The model under review builds one solid part; all positions refer to its coordinate system, in mm. A direction names the side the tool comes from. Give positions to 0.01 mm unless a question says otherwise; leave off trailing zeros. Order: outer loops, then holes, each group sorted by start corner. A loop starts at its lowest first (then second) coordinate and runs counter-clockwise, first axis right, second up. Notation, with made-up numbers: (-3.5, 83) - (48.5, 83) arc R19 ccw to (48.5, 92) - close; hole circle Ø10 at (22, -33). An arc over 180 degrees is marked (long way). Answer as CSV lines item,"result". Start each with the question number.
from build123d import *

# Parameters (mm, degrees)
F0_W     = 5
F0_H     = 95
F1_DEPTH = 1.4
F3_DEPTH = 8
F5_DEPTH = 111


with BuildPart() as f1:
    # F0 (on Top) → F1 (new body)
    with BuildSketch(Plane.XY):
        Polygon((86.25, 47.5), (86.25, 57.5), (-86.25, 57.5), (-86.25, -57.5), (86.25, -57.5), (86.25, -47.5), (53.75, -47.5), (48.75, -47.5), (-11.25, -47.5), (-16.25, -47.5), (-76.25, -47.5), (-76.25, 47.5), (-16.25, 47.5), (-11.25, 47.5), (48.75, 47.5), (53.75, 47.5), align=None)
        with Locations((-13.75, 0)):
            Rectangle(F0_W, F0_H)
        with Locations((51.25, 0)):
            Rectangle(F0_W, F0_H)
    extrude(amount=F1_DEPTH)

    # F2 (on face) → F3 (join)
    with BuildSketch(Plane.XY.offset(1.4)):
        Polygon((86.25, -57.5), (86.25, -55.5), (-84.25, -55.5), (-84.25, 55.5), (86.25, 55.5), (86.25, 57.5), (-86.25, 57.5), (-86.25, -57.5), align=None)
    extrude(amount=F3_DEPTH)

    # F4 (on face) → F5 (join, through all)
    with BuildSketch(Plane.XZ.offset(-55.5)):
        Polygon((-84.25, 9.4), (-84.25, 7.737799), (-82.629912, 9.4), align=None)
    extrude(amount=F5_DEPTH)


solid = f1.part
Item 1: Take a section at A-A on y = -9. Write out the cut boundary in (x, z).
Item 2: Machinability: for faces 4 (the face through (-13, -4, 0)), 5 (the face through (-84.25, -1, 5)), which of the approach directions +Z, -Z, +X, -X, +Y, -Y give a long, thin tool a straight path to every point of the face, cutting with its end or side? Answer none if there is none.
Item 3: Take a section at C-C on z = 6. Write out the cut boundary in (x, y).
Item 4: Take a section at B-B on x = 61. Write out the cut boundary in (y, z), and give its area (3 significant figures).
Item 5: Clearance check with flat-ended pins moving along their axes: pin 1 (3 mm diameter, centred on y = -37.5, z = 5.5, fed in from +X); pin 2 (1.1 mm diameter, centred on y = 15, z = 1, fed in from +X); pin 3 (12 mm diameter, centred on x = -34.5, y = -43.5, fed in from +Z). State where each tip first meets the part, or that it passes through.
Item 6: For line 1 along X through (y, z) = (31, 0.5); line 2 along Y through (x, z) = (-64.5, 2.25); line 3 along X through (y, z) = (-9, 5.25), list the stretches that pass through material, from the lowest coordinate up.
Item 7: Mouldability with a two-part tool opening along Y and no side actions: class faces 1 (the face through (2, -55.5, 5)), 2 (the face through (-38, 56, 9.4)), 3 (the face through (-1, -57.5, 5)) as released by +Y, released by -Y, zero draft, split by the parting line, or undercut.
Data:
1,outline,"(-86.25, 0) - (-76.25, 0) - (-76.25, 1.4) - (-84.25, 1.4) - (-84.25, 7.74) - (-82.63, 9.4) - (-86.25, 9.4) - close; (-16.25, 0) - (-11.25, 0) - (-11.25, 1.4) - (-16.25, 1.4) - close; (48.75, 0) - (53.75, 0) - (53.75, 1.4) - (48.75, 1.4) - close"
2,face 4,"-Z, +X, -X, +Y, -Y"
2,face 5,"+X"
3,outline,"(-86.25, -57.5) - (86.25, -57.5) - (86.25, -55.5) - (-84.25, -55.5) - (-84.25, 55.5) - (86.25, 55.5) - (86.25, 57.5) - (-86.25, 57.5) - close"
4,outline,"(-57.5, 0) - (-47.5, 0) - (-47.5, 1.4) - (-55.5, 1.4) - (-55.5, 9.4) - (-57.5, 9.4) - close; (47.5, 0) - (57.5, 0) - (57.5, 9.4) - (55.5, 9.4) - (55.5, 1.4) - (47.5, 1.4) - close"
4,area,"60.0 mm^2"
5,pin 1,"stops at x = -84.25"
5,pin 2,"stops at x = 53.75"
5,pin 3,"stops at z = 1.4"
6,line 1,"x = -86.25 to -76.25, -16.25 to -11.25, 48.75 to 53.75"
6,line 2,"y = -57.5 to -55.5, 55.5 to 57.5"
6,line 3,"x = -86.25 to -84.25"
7,face 1,"undercut"
7,face 2,"zero draft"
7,face 3,"released by -Y"
